Geometry: see drawing. Coordinates: mm, zero at the bounding-box minimum. Give positions to 0.01 mm unless a question says otherwise; leave off trailing zeros. Order: outer loops, then holes, each group sorted by start corner. A loop starts at its lowest first (then second) coordinate and runs counter-clockwise, first axis right, second up. Notation, with made-up numbers: M 81.5,86 L 111.5,86 A19 ccw 111.5,122 Z; hole C 22.25,83 d6. An arc over 180 degrees is marked long. Answer as a JSON object with one key per item and string values. Group by question number.
1. Section query A-A (z = 2.2). Output: boundary loops of the cut face in (x, y).
2. Material intervals for L1, parallel to Y at x = 155, z = 2.35; L2, parallel to Y at x = 36, z = 0.4; L3, parallel to Y at x = 158, z = 2, sorted ascending. Write a range as [from, to].
3. Pin query (flat end, axial travel): P1, Ø0.9, axis at y = 9.5, z = 1.5, coming from the +X side; P2, Ø1.5, axis at x = 155.5, z = 2, coming from the -Y side; P3, Ø2.5, axis at x = 6, y = 6, coming from the +Z side. Return the tip coordinate at first contact, or that it passes through.
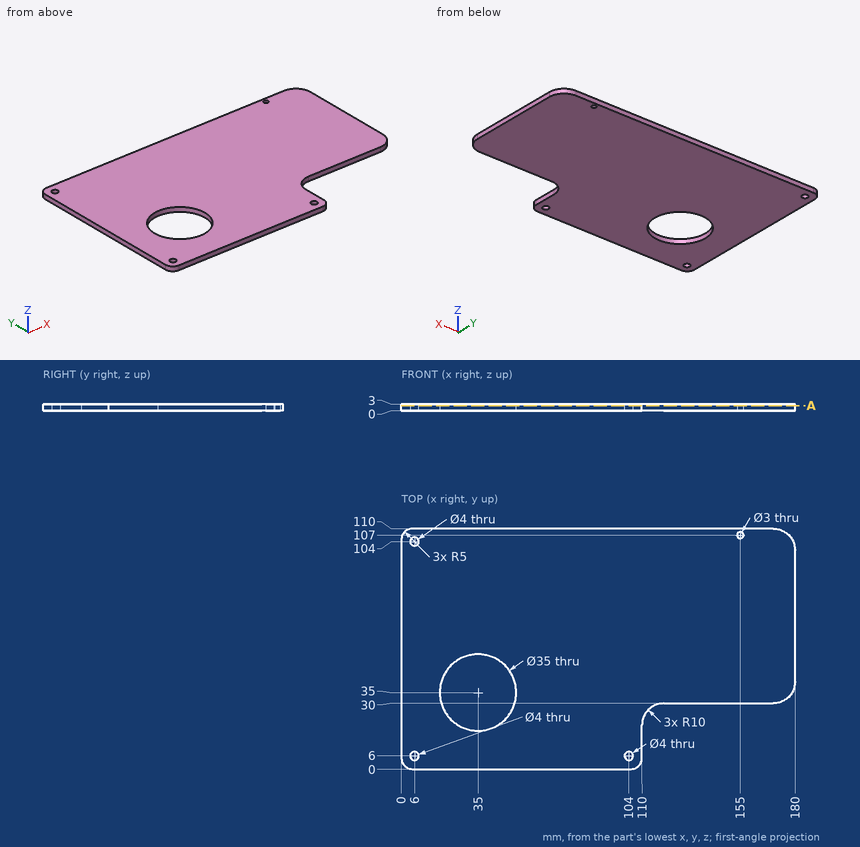
Answer sheet:
{
 "1": {"outline": "M 0,5 A5 ccw 5,0 L 105,0 A5 ccw 110,5 L 110,20 A10 cw 120,30 L 170,30 A10 ccw 180,40 L 180,100 A10 ccw 170,110 L 5,110 A5 ccw 0,105 Z; hole C 6,6 d4; hole C 6,104 d4; hole C 35,35 d35; hole C 104,6 d4; hole C 155,107 d3"},
 "2": {"L1": "[30, 105.5], [108.5, 110]", "L2": "[0, 17.53], [52.47, 110]", "L3": "[30, 110]"},
 "3": {"P1": "x = 110", "P2": "y = 30", "P3": "through"}
}
